```python
from build123d import *

# Parameters (mm, degrees)
F0_R     = 13.49375
F1_DEPTH = 25.4
F2_R     = 13.49375
F3_DEPTH = 25.4
F5_R     = 11.1506
F6_DEPTH = 46.736
F7_R     = 11.1506
F8_DEPTH = 50.8
F4_R     = 13.49375


with BuildPart() as f1:
    # F0 (on Right) → F1 (new body)
    with BuildSketch(Plane.YZ):
        with Locations((-15.2131393552, 0)):
            Circle(F0_R)
    extrude(amount=F1_DEPTH)

    # F5 (on face) → F6 (cut)
    with BuildSketch(Plane.YZ.offset(25.4)):
        with Locations((-15.2131393552, 0)):
            Circle(F5_R)
    extrude(amount=-F6_DEPTH, mode=Mode.SUBTRACT)



with BuildPart() as f3:
    # F2 (on Front) → F3 (new body)
    with BuildSketch(Plane.XZ):
        with Locations((-16.4639353752, 0)):
            Circle(F2_R)
    extrude(amount=-F3_DEPTH)

    # F7 (on face) → F8 (cut)
    with BuildSketch(Plane(origin=(0, 25.4, 0), x_dir=(-1, 0, 0), z_dir=(0, 1, 0))):
        with Locations((16.4639353752, 0)):
            Circle(F7_R)
    extrude(amount=-F8_DEPTH, mode=Mode.SUBTRACT)


with BuildPart() as f1_1:
    add(f1.part)

    add(f3.part)  # F10 merges F3
    # F10: sweep along a path in F9
    with BuildLine(Plane.XY) as f10_path:
        ThreePointArc((-30.3589254618, 0), (-18.8559760564, -18.1880432135), (0, -28.5598766059))
    # F4 (on face) → F10 (sweep)
    with BuildSketch(Plane.XZ):
        with Locations((-16.4639353752, 0)):
            Circle(F4_R)
    sweep(path=f10_path.line)


solid = f1_1.part
```
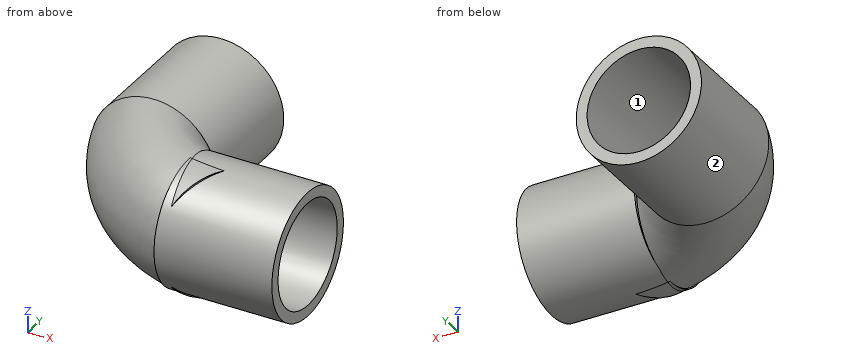
The listing builds one solid part. Answer for the finished solid, in the listing's coordinates (mm). Face numbers are marked on the shaded views. Give positions to 0.01 mm unless a question says otherwise; leave off trailing zeros. Order: outer loops, then holes, each group sorted by start corner. A loop starts at its lowest first (then second) coordinate and runs counter-clockwise, first axis right, second up.
Item 1: Find the intervals of material crossed by probe 1 along X at (y, z) = (17, -0.25); probe 2 along Y at (x, z) = (5.5, -3); probe 3 along Y at (x, z) = (19, 0), in increasing order.
From the geometry:
probe 1: x = -29.96 to -27.61, -5.32 to -2.97
probe 2: y = -28.37 to -25.95, -19.84 to -5.33, -4.47 to -2.06
probe 3: y = -28.71 to -26.36, -4.06 to -1.72
Item 2: The part is cut by section B-B, the plane x = 9.5. Count the separate pieces of the cut face and the enclosed holes in it, and give its area (3 significant figures).
From the geometry:
separate pieces: 1
enclosed holes: 2
area: 318 mm2
Item 3: The part is cut by section A-A, the plane y = 11. Give the vertices of the cut face in (x, z).
From the geometry:
outline: circle Ø26.99 at (-16.46, 0); hole circle Ø22.3 at (-16.46, 0)
Item 4: Given pin 1 Ø1 at (y, z) = (-13, 0) entering from +X; pin 2 Ø1 at (x, z) = (-4, 8.5) entering from +Y; pin 3 Ø10.5 at (y, z) = (-8.5, 4) entering from -X, each flat-ended and moving along its own axis, determine where each tip first touches the part or whether it passes through.
From the geometry:
pin 1: stops at x = 10.13
pin 2: stops at y = -1.52
pin 3: stops at x = -28.43
Item 5: For a pull along X with two mould halves and no side action, classify the marked faces 1 and 2 as pulls with the +X half, pulls with the -X half, needs draft (parallel to the pull), parting line crosses it, or undercut.
From the geometry:
face 1: undercut
face 2: parting line crosses it
